For this review, take the finished solid that the model builds, in its own axes (mm). Face numbers are marked on the shaded views. Give positions to 0.01 mm unless a question says otherwise; leave off trailing zeros. Order: outer loops, then holes, each group sorted by start corner. A loop starts at its lowest first (then second) coordinate and runs counter-clockwise, first axis right, second up. Notation, with made-up numbers: (-4, 59) - (2, 59) arc R15 cw to (2, 66) - close; hole circle Ø8 at (13, -0.75). An arc over 180 degrees is marked (long way). One line per item, written item: value.
```python
from build123d import *

# Parameters (mm, degrees)
SKETCH1_W               = 122
SKETCH1_H               = 108
BOSS_EXTRUDE1_DEPTH     = 11
SKETCH4_W               = 116
SKETCH4_H               = 102
CUT_EXTRUDE1_DEPTH      = 8
SKETCH6_R               = 1.999999993
SKETCH6_R_2             = 2
CUT_EXTRUDE6_DEPTH      = 120
CUT_EXTRUDE6_DEPTH_BACK = 4
SKETCH5_R               = 2
CUT_EXTRUDE5_DEPTH      = 106
CUT_EXTRUDE5_DEPTH_BACK = 4
FILLET2_R               = 1


with BuildPart() as part:
    # Sketch1 → Boss-Extrude1 (new body)
    with BuildSketch(Plane(origin=(0, 0, 0), x_dir=(1, 0, 0), z_dir=(0, 1, 0))):
        with Locations((-140.609907121, 23.894736842)):
            Rectangle(SKETCH1_W, SKETCH1_H)
    extrude(amount=BOSS_EXTRUDE1_DEPTH)

    # Sketch4 → Cut-Extrude1 (cut)
    with BuildSketch(Plane(origin=(0, 11, 0), x_dir=(1, 0, 0), z_dir=(0, 1, 0))):
        with Locations((-140.609907121, 23.894736842)):
            Rectangle(SKETCH4_W, SKETCH4_H)
    extrude(amount=-CUT_EXTRUDE1_DEPTH, mode=Mode.SUBTRACT)

    # Sketch6 → Cut-Extrude6 (cut, two sides)
    with BuildSketch(Plane(origin=(-198.609907121, 0, 0), x_dir=(0, 0, -1), z_dir=(1, 0, 0))) as cut_extrude6_sk:
        with Locations((-1.105263158, 6.999999977)):
            Circle(SKETCH6_R)
        with Locations((23.894736842, 6.999999988)):
            Circle(SKETCH6_R)
        with Locations((48.894736842, 7)):
            Circle(SKETCH6_R_2)
    extrude(amount=CUT_EXTRUDE6_DEPTH, mode=Mode.SUBTRACT)
    extrude(cut_extrude6_sk.sketch, amount=-CUT_EXTRUDE6_DEPTH_BACK, mode=Mode.SUBTRACT)

    # Sketch5 → Cut-Extrude5 (cut, two sides)
    with BuildSketch(Plane.XY.offset(-74.894736842)) as cut_extrude5_sk:
        with Locations((-169.359907121, 7)):
            Circle(SKETCH5_R)
        with Locations((-140.109907121, 7)):
            Circle(SKETCH5_R)
        with Locations((-110.859907121, 7)):
            Circle(SKETCH5_R)
    extrude(amount=CUT_EXTRUDE5_DEPTH, mode=Mode.SUBTRACT)
    extrude(cut_extrude5_sk.sketch, amount=-CUT_EXTRUDE5_DEPTH_BACK, mode=Mode.SUBTRACT)

    # Fillet2
    fillet2_edges = [part.edges().sort_by_distance(p)[0] for p in [
        (-79.609907121, 11, -23.894736842),
        (-140.609907121, 11, -77.894736842),
        (-198.609907121, 11, -23.894736842),
        (-140.609907121, 11, 27.105263158),
        (-82.609907121, 11, -23.894736842),
        (-140.609907121, 11, -74.894736842),
        (-201.609907121, 11, -23.894736842),
        (-140.609907121, 11, 30.105263158),
    ]]
    fillet(fillet2_edges, radius=FILLET2_R)


solid = part.part
```
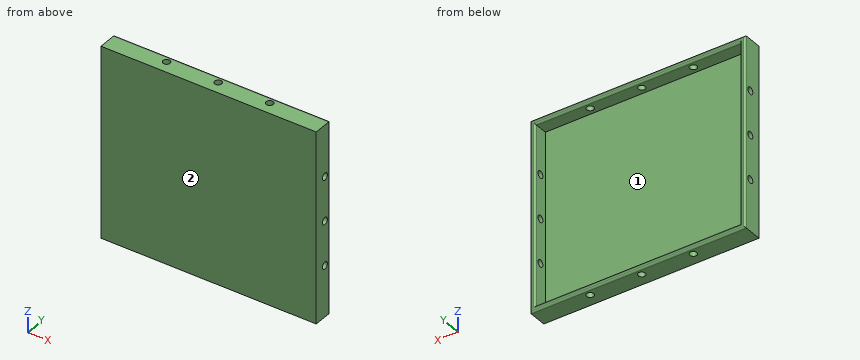
(1) Draft analysis for pull direction Z (two halves, no side actions). For the marked faces 1 and 2, state which applies: pulls with the +Z half, pulls with the -Z half, needs draft (parallel to the pull), parting line crosses it, or undercut.
Answers below:
face 1: undercut
face 2: needs draft
(2) Take a section at B-B (x = -160). Write out the cut boundary in (y, z).
Answers below:
outline: (0, -77.89) - (10, -77.89) arc R1 ccw to (11, -76.89) - (11, -75.89) arc R1 ccw to (10, -74.89) - (3, -74.89) - (3, 27.11) - (10, 27.11) arc R1 ccw to (11, 28.11) - (11, 29.11) arc R1 ccw to (10, 30.11) - (0, 30.11) - close
(3) Take a section at C-C (x = -139.5). Write out the cut boundary in (y, z).
Answers below:
outline: (0, -77.89) - (5.1, -77.89) - (5.1, -74.89) - (3, -74.89) - (3, 27.11) - (5.1, 27.11) - (5.1, 30.11) - (0, 30.11) - close; (8.9, -77.89) - (10, -77.89) arc R1 ccw to (11, -76.89) - (11, -75.89) arc R1 ccw to (10, -74.89) - (8.9, -74.89) - close; (8.9, 27.11) - (10, 27.11) arc R1 ccw to (11, 28.11) - (11, 29.11) arc R1 ccw to (10, 30.11) - (8.9, 30.11) - close
(4) Wall thickness on line 1 (X direction, y = 7, z = 28.2); line 2 (Z direction, x = -81.65, y = 7); line 3 (X direction, y = 10, z = -12): over which ranges is each line inside the solid? List them lowest first. Write a range as from..to.
Answers below:
line 1: x = -201.61..-171.36, -167.36..-142.11, -138.11..-112.86, -108.86..-79.61
line 2: z = -77.89..-50.89, -46.89..-25.89, -21.89..-0.89, 3.11..30.11
line 3: x = -201.61..-198.61, -82.61..-79.61
(5) Take a section at A-A (z = -67.5). Write out the cut boundary in (x, y).
Answers below:
outline: (-201.61, 0) - (-79.61, 0) - (-79.61, 10) arc R1 ccw to (-80.61, 11) - (-81.61, 11) arc R1 ccw to (-82.61, 10) - (-82.61, 3) - (-198.61, 3) - (-198.61, 10) arc R1 ccw to (-199.61, 11) - (-200.61, 11) arc R1 ccw to (-201.61, 10) - close
(6) For P1, Ø5, axis at y = 7, z = 1.11, coming from the -X side; P2, Ø10, axis at x = -186, z = -2.5, coming from the +Y side, all flat-tipped, find the tip position at first contact; note any pin that passes through.
Answers below:
P1: stops at x = -201.61
P2: stops at y = 3
